Can you work these out from the drawing? Everything is in mm from the part's minimum corner. A direction names the side the tool comes from. Round coordinates to 2 decimals unless told otherwise and drop trailing zeros. Write each loop counter-clockwise with the first axis right and the second up, starting at its lowest first coordinate (ties: lowest second). Pieces come first, ordered by that corner, then holes. Notation, with made-up numbers: (-31, -25.5) -> (15, -25.5) arc R17 cw to (15, -11.5) -> close; hole circle Ø6 at (-8.75, 78). An arc over 180 degrees is marked (long way). Put each result on its own line as item: value. Start each with the question number.
1. We'd pull the mould along X, two halves only. Please class the marked faces 4, 5 and 6: +X half, -X half, draft (parallel to the pull), parting line (faces both ways), or undercut.
2. Suppose I cut it at D-D (z = 12.7). Please give me the cut outline in (x, y) (3 decimals), then the cut area to 3 significant figures.
3. I need wall thicknesses on probe 1 along X at (y, z) = (2.45, 12.7); probe 2 along X at (y, z) = (3.25, 11.5); probe 3 along Z at (x, y) = (7.62, 1.5). Which ranges of each line are inside material? Lowest first, please. Write a range as from..to.
4. Which directions (+Z, -Z, +X, -X, +Y, -Y) give clear straight access to the entire face, cutting with the end or side of a thin tool? Please do the marked faces 1, 2 and 3.
5. Suppose I cut it at A-A (y = 2.25). Please give me the cut outline in (x, z), then the cut area to 3 significant figures.
6. For pin 1 (3 mm diameter, centred on x = 38, y = 10, fed in from -Z); pin 2 (6 mm diameter, centred on x = 26.5, z = 10, fed in from -Y); pin 3 (3.5 mm diameter, centred on y = 8, z = 13.5, fed in from +X); pin 4 (7.5 mm diameter, centred on x = 44.5, z = 19, fed in from +Y) (3 decimals), each with a flat end and sliding along its axis, tell me the tip position at first contact or that it passes through.
7. Suppose I cut it at B-B (y = 6). Please give me the cut outline in (x, z), then the cut area to 3 significant figures.
8. Suppose I cut it at C-C (x = 7.62). Please give me the cut outline in (y, z) (3 decimals).
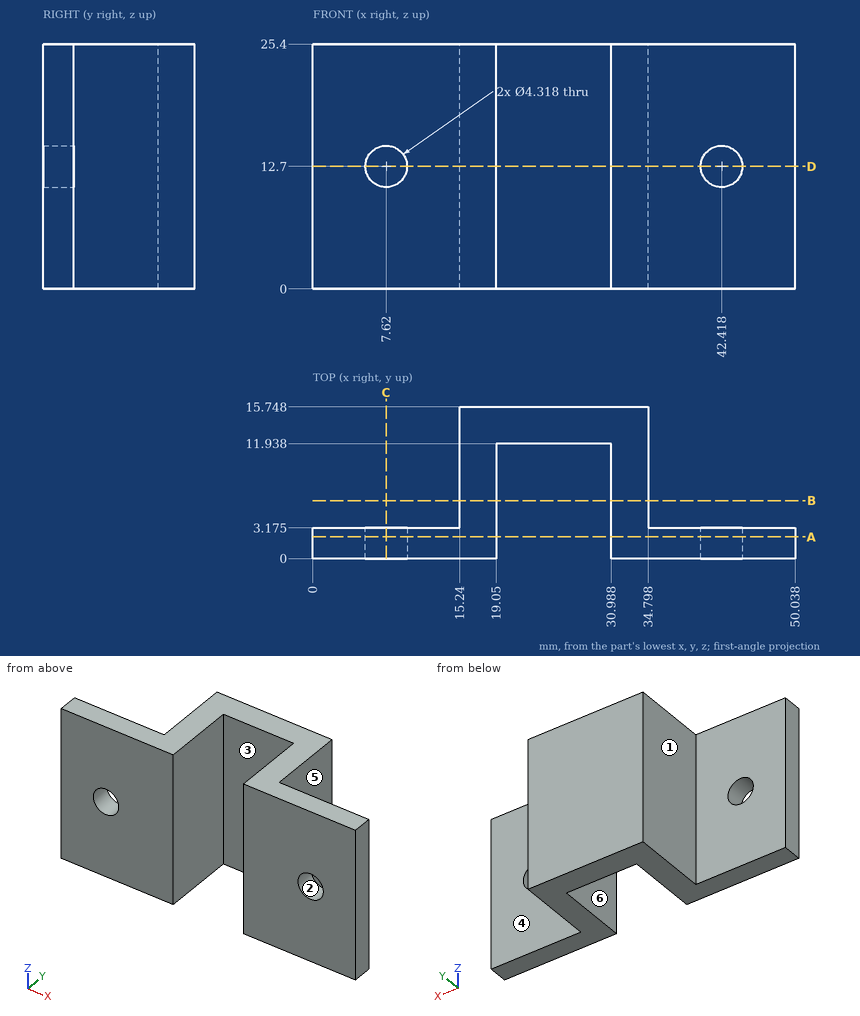
Verdict:
1. face 4: draft
1. face 5: +X half
1. face 6: undercut
2. outline: (0, 0) -> (5.461, 0) -> (5.461, 3.175) -> (0, 3.175) -> close; (9.779, 0) -> (19.05, 0) -> (19.05, 11.938) -> (30.988, 11.938) -> (30.988, 0) -> (40.259, 0) -> (40.259, 3.175) -> (34.798, 3.175) -> (34.798, 15.748) -> (15.24, 15.748) -> (15.24, 3.175) -> (9.779, 3.175) -> close; (44.577, 0) -> (50.038, 0) -> (50.038, 3.175) -> (44.577, 3.175) -> close
2. area: 235 mm^2
3. probe 1: x = 0..5.46, 9.78..19.05, 30.99..40.26, 44.58..50.04
3. probe 2: x = 15.24..19.05, 30.99..34.8
3. probe 3: z = 0..10.54, 14.86..25.4
4. face 1: +Z, -Z, -X, +Y
4. face 2: +Y, -Y
4. face 3: +Z, -Z, -Y
5. outline: (0, 0) -> (19.05, 0) -> (19.05, 25.4) -> (0, 25.4) -> close; (30.99, 0) -> (50.04, 0) -> (50.04, 25.4) -> (30.99, 25.4) -> close; hole circle Ø4.32 at (7.62, 12.7); hole circle Ø4.32 at (42.42, 12.7)
5. area: 938 mm^2
6. pin 1: passes through
6. pin 2: stops at y = 11.94
6. pin 3: stops at x = 34.8
6. pin 4: stops at y = 3.175
7. outline: (15.24, 0) -> (19.05, 0) -> (19.05, 25.4) -> (15.24, 25.4) -> close; (30.99, 0) -> (34.8, 0) -> (34.8, 25.4) -> (30.99, 25.4) -> close
7. area: 194 mm^2
8. outline: (0, 0) -> (3.175, 0) -> (3.175, 10.541) -> (0, 10.541) -> close; (0, 14.859) -> (3.175, 14.859) -> (3.175, 25.4) -> (0, 25.4) -> close
